The model under review builds one solid part; all positions refer to its coordinate system, in mm. Round coordinates to 2 decimals unless told otherwise and drop trailing zeros. Order: outer loops, then holes, each group sorted by start corner. A loop starts at its lowest first (then second) coordinate and runs counter-clockwise, first axis right, second up. Notation, with made-up numbers: (31.5, 28.5) -> (79.5, 28.5) arc R15 cw to (79.5, 42.5) -> close; hole circle Ø1 at (26, 5.25). An arc over 180 degrees is marked (long way). Use a Markdown table: item, result. Add a question column.
```python
from build123d import *

# Parameters (mm, degrees)
SKETCH3_W           = 6
SKETCH3_H           = 6
BOSS_EXTRUDE1_DEPTH = 6
SKETCH4_R           = 1
CUT_EXTRUDE1_DEPTH  = 6
CUT_EXTRUDE2_REACH  = 9.348
SKETCH5_R           = 1
FILLET1_R           = 1


with BuildPart() as part:
    # Sketch3 → Boss-Extrude1 (new body)
    with BuildSketch(Plane(origin=(0, 0, 0), x_dir=(1, 0, 0), z_dir=(0, 1, 0))):
        Rectangle(SKETCH3_W, SKETCH3_H)
    extrude(amount=BOSS_EXTRUDE1_DEPTH)

    # Sketch4 → Cut-Extrude1 (cut)
    with BuildSketch(Plane.XY.offset(3)):
        with Locations((0, 3)):
            Circle(SKETCH4_R)
    extrude(amount=-CUT_EXTRUDE1_DEPTH, mode=Mode.SUBTRACT)

    # Cut-Extrude2: up to this face of the body (flat: up to its plane)
    cut_extrude2_end = Plane(part.part.faces().sort_by_distance((0, 0, 0))[0])
    # Sketch5 → Cut-Extrude2 (cut, up to the picked face)
    with BuildSketch(Plane(origin=(0, 6, 0), x_dir=(1, 0, 0), z_dir=(0, 1, 0)), mode=Mode.PRIVATE) as cut_extrude2_sk1:
        with Locations(Location((0, 0, 0), (0, 0, 270))):
            Circle(SKETCH5_R)
    cut_extrude2_tool1 = split(extrude(cut_extrude2_sk1.sketch, amount=-CUT_EXTRUDE2_REACH, mode=Mode.PRIVATE), bisect_by=cut_extrude2_end, keep=Keep.BOTH, mode=Mode.PRIVATE)
    add(cut_extrude2_tool1.solids().sort_by(Axis((0, 6, 0), (0, -1, 0)))[0], mode=Mode.SUBTRACT)

    # Fillet1
    fillet1_edges = [part.edges().sort_by_distance(p)[0] for p in [
        (-3, 6, 0),
        (0, 6, 3),
        (3, 6, 0),
        (0, 0, 3),
        (-3, 0, 0),
        (0, 0, -3),
        (3, 0, 0),
        (3, 3, 3),
        (-3, 3, 3),
        (-3, 3, -3),
        (3, 3, -3),
        (0, 6, -3),
    ]]
    fillet(fillet1_edges, radius=FILLET1_R)


solid = part.part
```
Q1. Draft analysis for pull direction X (two halves, no side actions). For faces 1 (the face through (-2.715, 0.301, -0.028)), 2 (the face through (-1, 0, -1)), 3 (the face through (-1, 3, -2)), 4 (the face through (2.699, 3.028, 2.715)), state which applies: released by +X, released by -X, zero draft, split by the parting line, or undercut.
Q2. Add section C-C, the plane y = 3.6. Give the boundary of the cut face in (x, z).
Q3. Add section D-D, the plane x = -2.6. Give the boundary of the cut face in (y, z).
Q4. Add section A-A, the plane x = 0.8. Give the boundary of the cut face in (y, z).
Q5. Add section B-B, the plane z = 0.8. Give the boundary of the cut face in (x, y), then the cut area to 3 significant figures.
Q6. To check wall thickness, follow line 1 along X through (y, z) = (3, 1.8); line 2 along Y through (x, z) = (0, -1.4); line 3 along Y through (x, z) = (-0.9, -1). State the ranges of each line that lie inside material, in increasing order.
Return value:
| question | item | result |
|---|---|---|
| 1 | face 1 | released by -X |
| 1 | face 2 | zero draft |
| 1 | face 3 | undercut |
| 1 | face 4 | released by +X |
| 2 | outline | (-3, -2) arc R1 ccw to (-2, -3) -> (-0.8, -3) -> (-0.8, -0.6) arc R1 cw to (-0.8, 0.6) -> (-0.8, 3) -> (-2, 3) arc R1 ccw to (-3, 2) -> close; (0.8, -3) -> (2, -3) arc R1 ccw to (3, -2) -> (3, 2) arc R1 ccw to (2, 3) -> (0.8, 3) -> (0.8, 0.6) arc R1 cw to (0.8, -0.6) -> close |
| 3 | outline | (0.2, -2) arc R0.8 ccw to (1, -2.8) -> (5, -2.8) arc R0.8 ccw to (5.8, -2) -> (5.8, 2) arc R0.8 ccw to (5, 2.8) -> (1, 2.8) arc R0.8 ccw to (0.2, 2) -> close |
| 4 | outline | (0, -2) arc R1 ccw to (1, -3) -> (2.4, -3) -> (2.4, -0.6) -> (0, -0.6) -> close; (0, 0.6) -> (2.4, 0.6) -> (2.4, 3) -> (1, 3) arc R1 ccw to (0, 2) -> close; (3.6, -3) -> (5, -3) arc R1 ccw to (6, -2) -> (6, -0.6) -> (3.6, -0.6) -> close; (3.6, 0.6) -> (6, 0.6) -> (6, 2) arc R1 ccw to (5, 3) -> (3.6, 3) -> close |
| 5 | outline | (-3, 1) arc R1 ccw to (-2, 0) -> (-0.6, 0) -> (-0.6, 2.2) arc R1 cw to (-0.6, 3.8) -> (-0.6, 6) -> (-2, 6) arc R1 ccw to (-3, 5) -> close; (0.6, 0) -> (2, 0) arc R1 ccw to (3, 1) -> (3, 5) arc R1 ccw to (2, 6) -> (0.6, 6) -> (0.6, 3.8) arc R1 cw to (0.6, 2.2) -> close |
| 5 | area | 27.0 mm² |
| 6 | line 1 | -3 to -1, 1 to 3 |
| 6 | line 2 | 0 to 2, 4 to 6 |
| 6 | line 3 | 0 to 2.56, 3.44 to 6 |
